from build123d import *

# Parameters (mm, degrees)
SKETCH2_W           = 150
SKETCH2_H           = 100
BOSS_EXTRUDE1_DEPTH = 10


with BuildPart() as part:
    # Sketch2 → Boss-Extrude1 (new body)
    with BuildSketch(Plane.XY):
        Rectangle(SKETCH2_W, SKETCH2_H)
        Polygon((0, -35.355339059), (35.355339059, 0), (0, 35.355339059), (-35.355339059, 0), align=None, mode=Mode.SUBTRACT)
    extrude(amount=BOSS_EXTRUDE1_DEPTH)


solid = part.part
The listing builds one solid part. Answer for the finished solid, in the listing's coordinates (mm). A direction names the side the tool comes from. Coordinates: 2 decimals unless noted, no trailing zeros. Order: outer loops, then holes, each group sorted by start corner. A loop starts at its lowest first (then second) coordinate and runs counter-clockwise, first axis right, second up.
Q1. For a pull along Y with two mould halves and no side action, classify faces 3 (the face through (-1, 50, 5)), 4 (the face through (17.43, -17.925, 4.93)), 5 (the face through (-75, -1, 5)), 6 (the face through (17.925, 17.43, 4.93)) as pulls with the +Y half, pulls with the -Y half, needs draft (parallel to the pull), parting line crosses it, or undercut.
Q2. A cutting plane is placed at A-A, the plane z = 3.25. Write down the section's boundary in (x, y), and give its area (3 significant figures).
Q3. Consider line 1 (Y direction, x = 0, z = 8.25); line 2 (X direction, y = 29, z = 2.75); line 3 (X direction, y = 10, z = 9). Determine where each line is inside the solid, lowest interval first.
Q4. A cutting plane is placed at C-C, the plane x = -16. Write down the section's boundary in (y, z), and give its area (3 significant figures).
Q5. A cutting plane is placed at B-B, the plane y = 3.5. Write down the section's boundary in (x, z), and give its area (3 significant figures).
Q6. Which of the six approach directions +Z, -Z, +X, -X, +Y, -Y give full straight-line access (tool end or side, diameter ignored) to faces 1 (the face through (-18, 23, 10)), 2 (the face through (-17.43, 17.925, 4.93))?
Answers follow:
1. face 3: pulls with the +Y half
1. face 4: undercut
1. face 5: needs draft
1. face 6: undercut
2. outline: (-75, -50) - (75, -50) - (75, 50) - (-75, 50) - close; hole (-35.36, 0) - (0, -35.36) - (35.36, 0) - (0, 35.36) - close
2. area: 12,500 mm2
3. line 1: y = -50 to -35.36, 35.36 to 50
3. line 2: x = -75 to -6.36, 6.36 to 75
3. line 3: x = -75 to -25.36, 25.36 to 75
4. outline: (-50, 0) - (-19.36, 0) - (-19.36, 10) - (-50, 10) - close; (19.36, 0) - (50, 0) - (50, 10) - (19.36, 10) - close
4. area: 613 mm2
5. outline: (-75, 0) - (-31.86, 0) - (-31.86, 10) - (-75, 10) - close; (31.86, 0) - (75, 0) - (75, 10) - (31.86, 10) - close
5. area: 863 mm2
6. face 1: +Z, +X, -X, +Y, -Y
6. face 2: +Z, -Z
